The model under review builds one solid part; all positions refer to its coordinate system, in mm. Round coordinates to 2 decimals unless told otherwise and drop trailing zeros. Loops run counter-clockwise (first coordinate to the right, second up) from the corner with the lowest first, then second, coordinate; pieces in that order, holes last. Notation, with made-up numbers: (59, -5.75) -> (80, -5.75) arc R22 ccw to (80, 11.25) -> close; hole circle Ø11 at (1.25, 82). An arc over 180 degrees is marked (long way). Write each question's results on one line, items separated by ' | '. Start each with the question number.
Item 1: Clearance check with a flat-ended pin moving along its axis: pin 1 Ø5.5 at (x, y) = (11.46, -8.75) entering from +Z. State where the tip first meets the part, or that it passes through.
Item 2: Mouldability with a two-part tool opening along X and no side actions: class faces 1 (the flat face through (29, -16.749, 1)), 2 (the cylindrical face through (2.37, 28.4, 1.48)), 3 (the cylindrical face through (56.11, 28.35, 1.48)), 4 (the cylindrical face through (51.52, 22.74, 1.48)) as pulls with the +X half, pulls with the -X half, needs draft (parallel to the pull), parting line crosses it, or undercut.
Item 3: We need section A-A (z = 0.55). Give the boundary of the cut face in (x, y), and give its area (3 significant figures).
Item 4: For L1, parallel to Y at x = 51.5, z = 1.65; L2, parallel to X at y = -8, z = 0.5; L3, parallel to Y at x = 11.5, z = 2.75, list the stretches that pass through material, from the lowest coordinate up. Write a range as from..to.
from build123d import *

# Parameters (mm, degrees)
SKETCH_1_R      = 1.5
SKETCH_1_R_2    = 3
EXTRUDE_1_DEPTH = 3


with BuildPart() as part:
    # 草图1 → 凸台-拉伸1 (new body)
    with BuildSketch(Plane.XY):
        with BuildLine():
            Line((56.964417519, -13.748620871), (56.964417519, 26.251379129))
            ThreePointArc((56.964417519, 26.251379129), (56.085737863, 28.372699472), (53.964417519, 29.251379129))
            Line((53.964417519, 29.251379129), (4.464417519, 29.251379129))
            ThreePointArc((4.464417519, 29.251379129), (2.343097176, 28.372699472), (1.464417519, 26.251379129))
            Line((1.464417519, 26.251379129), (1.464417519, -13.748620871))
            ThreePointArc((1.464417519, -13.748620871), (2.343097176, -15.869941215), (4.464417519, -16.748620871))
            Line((4.464417519, -16.748620871), (53.964417519, -16.748620871))
            ThreePointArc((53.964417519, -16.748620871), (56.085737863, -15.869941215), (56.964417519, -13.748620871))
        make_face()
        with Locations((51.714417519, 21.251379129)):
            Circle(SKETCH_1_R, mode=Mode.SUBTRACT)
        with Locations((26.714417519, 21.251379129)):
            Circle(SKETCH_1_R, mode=Mode.SUBTRACT)
        with Locations(Location((26.714417519, -8.748620871, 0), (0, 0, 180))):
            Circle(SKETCH_1_R, mode=Mode.SUBTRACT)
        with Locations(Location((51.714417519, -8.748620871, 0), (0, 0, 180))):
            Circle(SKETCH_1_R, mode=Mode.SUBTRACT)
        with Locations((11.464417519, 21.251379129)):
            Circle(SKETCH_1_R_2, mode=Mode.SUBTRACT)
        with Locations(Location((11.464417519, -8.748620871, 0), (0, 0, 180))):
            Circle(SKETCH_1_R_2, mode=Mode.SUBTRACT)
    extrude(amount=EXTRUDE_1_DEPTH)


solid = part.part
Here are the results:
1) pin 1: passes through
2) face 1: needs draft | face 2: pulls with the -X half | face 3: pulls with the +X half | face 4: undercut
3) outline: (1.46, -13.75) arc R3 ccw to (4.46, -16.75) -> (53.96, -16.75) arc R3 ccw to (56.96, -13.75) -> (56.96, 26.25) arc R3 ccw to (53.96, 29.25) -> (4.46, 29.25) arc R3 ccw to (1.46, 26.25) -> close; hole circle Ø6 at (11.46, -8.75); hole circle Ø6 at (11.46, 21.25); hole circle Ø3 at (26.71, -8.75); hole circle Ø3 at (26.71, 21.25); hole circle Ø3 at (51.71, -8.75); hole circle Ø3 at (51.71, 21.25) | area: 2,460 mm2
4) L1: y = -16.75..-10.23, -7.26..19.77, 22.74..29.25 | L2: x = 1.46..8.56, 14.37..25.41, 28.01..50.41, 53.01..56.96 | L3: y = -16.75..-11.75, -5.75..18.25, 24.25..29.25
